from build123d import *

# Parameters (mm, degrees)
CROQUIS2_R              = 2.55
CROQUIS2_R_2            = 3.75
CROQUIS2_R_3            = 1.225
SALIENTE_EXTRUIR1_DEPTH = 75.8075
CORTAR_EXTRUIR1_DEPTH   = 101.016875761
CROQUIS5_W              = 71.8075
CROQUIS5_H              = 13
CORTAR_EXTRUIR2_DEPTH   = 101.016875761
REDONDEO1_R             = 2
CHAFL_N1_SIZE           = 5
CHAFL_N1_SIZE2          = 5.533110727
REDONDEO2_R             = 12
CORTAR_EXTRUIR3_DEPTH   = 91.170863593
REDONDEO3_R             = 12
REDONDEO4_R             = 6


with BuildPart() as part:
    # Croquis2 → Saliente-Extruir1 (new body)
    with BuildSketch(Plane.XY):
        with BuildLine():
            Line((-20, 31.5422), (-20, -6))
            Line((-20, -6), (20, -6))
            Line((20, -6), (20, 31.5422))
            ThreePointArc((20, 31.5422), (14.142135624, 45.684335624), (0, 51.5422))
            ThreePointArc((0, 51.5422), (-14.142135624, 45.684335624), (-20, 31.5422))
        make_face()
        with Locations(Location((-7.5, 0, 0), (0, 0, 180))):
            Circle(CROQUIS2_R, mode=Mode.SUBTRACT)
        with Locations(Location((7.5, 0, 0), (0, 0, 180))):
            Circle(CROQUIS2_R, mode=Mode.SUBTRACT)
        with Locations(Location((0, 40.6, 0), (0, 0, 180))):
            Circle(CROQUIS2_R_2, mode=Mode.SUBTRACT)
        with Locations(Location((0, 48.0422, 0), (0, 0, 180))):
            Circle(CROQUIS2_R_3, mode=Mode.SUBTRACT)
        with Locations(Location((0, 33.1578, 0), (0, 0, 180))):
            Circle(CROQUIS2_R_3, mode=Mode.SUBTRACT)
    extrude(amount=SALIENTE_EXTRUIR1_DEPTH)

    # Croquis4 → Cortar-Extruir1 (cut, through all)
    with BuildSketch(Plane.ZY.offset(20)):
        Polygon((0, 12), (70, 12), (71.8075, 31.5422), (71.8075, 53.713147715), (0, 53.713147715), align=None)
    extrude(amount=-CORTAR_EXTRUIR1_DEPTH, mode=Mode.SUBTRACT)

    # Croquis5 → Cortar-Extruir2 (cut, through all)
    with BuildSketch(Plane.ZY.offset(20)):
        with Locations((39.90375, 0.5)):
            Rectangle(CROQUIS5_W, CROQUIS5_H)
    extrude(amount=-CORTAR_EXTRUIR2_DEPTH, mode=Mode.SUBTRACT)

    # Redondeo1
    redondeo1_edges = [part.edges().sort_by_distance(p)[0] for p in [
        (0, 7, 4),
    ]]
    fillet(redondeo1_edges, radius=REDONDEO1_R)

    # Chaflán1
    chafl_n1_edges = [part.edges().sort_by_distance(p)[0] for p in [
        (0, 12, 70),
    ]]
    chafl_n1_side = [part.faces().sort_by_distance(p)[0] for p in [
        (0, 12, 35),
    ]]
    chamfer(chafl_n1_edges, length=CHAFL_N1_SIZE, length2=CHAFL_N1_SIZE2, reference=chafl_n1_side[0])

    # Redondeo2
    redondeo2_edges = [part.edges().sort_by_distance(p)[0] for p in [
        (20, -6, 2),
        (-20, -6, 2),
    ]]
    fillet(redondeo2_edges, radius=REDONDEO2_R)

    # Croquis7 → Cortar-Extruir3 (cut, through all)
    with BuildSketch(Plane.XZ.offset(-7)):
        Polygon((-20, 6), (-6.5, 15), (-6.5, 75.8075), (-20, 75.8075), align=None)
        Polygon((20, 75.8075), (20, 6), (6.5, 15), (6.5, 75.8075), align=None)
    extrude(amount=-CORTAR_EXTRUIR3_DEPTH, mode=Mode.SUBTRACT)

    # Redondeo3
    # the kernel refuses this fillet: 12 mm, written as the material it adds along each edge
    with BuildSketch(Plane(origin=(-6.5, 7, 15), x_dir=(-0.8320502943378436, 0, -0.5547001962252291), z_dir=(0, 1, 0)), Plane(origin=(6.5, 7, 15), x_dir=(0, 0, 1), z_dir=(0, 1, 0))) as redondeo3_piece_1:
        with BuildLine():
            CenterArc((REDONDEO3_R * 0.535183758488, REDONDEO3_R), REDONDEO3_R, 213.690067526, 56.309932474)
            Line((-REDONDEO3_R * 0.29686653585, REDONDEO3_R * 0.445299803775), (0, 0))
            Line((0, 0), (REDONDEO3_R * 0.535183758488, 0))
        make_face()
    extrude(amount=5)
    # the kernel refuses this fillet: 12 mm, written as the material it takes off along each edge
    with BuildSketch(Plane(origin=(20, -9.032649504, 6), x_dir=(0, 0, -1), z_dir=(0, 1, 0))) as redondeo3_2_piece_1:
        with BuildLine():
            CenterArc((6.427278002, 11.99239065), REDONDEO3_R, 213.690067526, 54.269398965)
            Line((-3.55732553, 5.335988296), (0, 0))
            Line((0, 0), (6, 0))
        make_face()
    extrude(amount=37.065299008, mode=Mode.SUBTRACT)
    with BuildSketch(Plane(origin=(-20, -9.032649504, 6), x_dir=(0, 0, -1), z_dir=(0, 1, 0))) as redondeo3_2_piece_2:
        with BuildLine():
            CenterArc((6.427278002, -11.99239065), REDONDEO3_R, 92.040533509, 54.269398965)
            Line((-3.55732553, -5.335988296), (0, 0))
            Line((0, 0), (6, 0))
        make_face()
    extrude(amount=37.065299008, mode=Mode.SUBTRACT)

    # Redondeo4
    redondeo4_edges = [part.edges().sort_by_distance(p)[0] for p in [
        (0, 7, 75.8075),
    ]]
    fillet(redondeo4_edges, radius=REDONDEO4_R)


solid = part.part
Check sheet for the modelled part. Datum: model origin and axes. Units: mm. A direction names the side the tool comes from. Round coordinates to 2 decimals unless told otherwise and drop trailing zeros. Loops run counter-clockwise (first coordinate to the right, second up) from the corner with the lowest first, then second, coordinate; pieces in that order, holes last. Notation, with made-up numbers: (4.5, -12.75) - (8.5, -12.75) arc R25 cw to (8.5, 2.25) - close; hole circle Ø3 at (28, 41). An arc over 180 degrees is marked (long way). Answer as CSV lines item,"result". Start each with the question number.
Item 1: Section check A-A (y = 0). Record the boundary of the cut face in (x, z), and give its area (3 significant figures).
Item 2: Section check B-B (x = -13). Record the boundary of the cut face in (y, z).
Item 3: Set-up check for faces 1 (the flat face through (-1, 7, 34)), 2 (the flat face through (6.5, 9, 59)), 3 (the cylindrical face through (-9.93, -0.77, 1.97)), 4 (the cylindrical face through (-14.991, -3.754, 2.028)), 5 (the flat face through (-1, 12, 24)): record each of +Z, -Z, +X, -X, +Y, -Y from which the full face is reachable in a straight line by a thin tool's end or side.
Item 4: Section check D-D (y = 20). Record the boundary of the cut face in (x, z), and give its area (3 significant figures).
Item 5: Scan lines: line 1 (X direction, y = 40.6, z = 74.35); line 2 (Z direction, x = 1.5, y = 0.5); line 3 (Y direction, x = 6, z = 64). Record each from-to range of solid material in increasing order. Write a range as [from, to].
Item 6: Depth check by flat-ended pin: P1, Ø12, axis at x = 0, y = 40.6, coming from the +Z side; P2, Ø12, axis at x = 12.5, z = 11.5, coming from the +Y side; P3, Ø12, axis at x = 0, z = 62.5, coming from the +Y side; P4, Ø14.5, axis at x = 0.5, y = 45, coming from the -Z side. Enter the tip coordinate at first touch or a pass-through.
Item 7: Release check for a two-part mould opening along X. For faces 6 (the cylindrical face through (0.09, 8.71, 74)), 7 (the cylindrical face through (0.488, 36.882, 73.78)), 8 (the cylindrical face through (14.774, -3.905, 2.028)), 9 (the cylindrical face through (-7.9, 9.5, 15.8)) record: +X half, -X half, draft (parallel to the pull), parting line (faces both ways), or undercut.
Item 8: Section check C-C (z = 33.5). Record the boundary of the cut face in (x, y).
Report:
1,outline,"(-18.39, 0) - (-10.05, 0) - (-10.05, 4) - (-18.39, 4) - close; (-4.95, 0) - (4.95, 0) - (4.95, 4) - (-4.95, 4) - close; (10.05, 0) - (18.39, 0) - (18.39, 4) - (10.05, 4) - close"
1,area,"106 mm2"
2,outline,"(-4.91, 0) - (12, 0) - (12, 10.67) - (7, 10.67) - (7, 6) arc R2 cw to (5, 4) - (-4.91, 4) - close"
3,face 1,"+Z, +X, -X, -Y"
3,face 2,"+Z, +X, +Y, -Y"
3,face 3,"+Z, -Z"
3,face 4,"+Z, -Z, -X, -Y"
3,face 5,"-Z, +X, -X, +Y"
4,outline,"(-6.5, 70.74) - (6.5, 70.74) - (6.5, 75.81) - (-6.5, 75.81) - close"
4,area,"65.9 mm2"
5,line 1,"x = [-6.5, -3.75], [3.75, 6.5]"
5,line 2,"z = [0, 4]"
5,line 3,"y = [7, 12]"
6,P1,"stops at z = 75.81"
6,P2,"stops at y = 12"
6,P3,"stops at y = 15.5"
6,P4,"stops at z = 71.81"
7,face 6,"draft"
7,face 7,"undercut"
7,face 8,"+X half"
7,face 9,"-X half"
8,outline,"(-6.5, 7) - (6.5, 7) - (6.5, 12) - (-6.5, 12) - close"
